```python
from build123d import *

# Parameters (mm, degrees)
F0_W     = 16.6126135737
F0_H     = 3.81
F0_W_2   = 7.62
F0_H_2   = 7.62
F1_DEPTH = 3.175


# Not quite as in the source:
# - a length typed as a fraction of an inch, garbled in the dataset ("3 / 203.2 mm" for 3/8 in), is restored
# - a feature names something its author has since deleted; it is built from what else it names


with BuildPart() as f1:
    # F0 (on Top) → F1 (new body)
    with BuildSketch(Plane.XY):
        Polygon((24.765, -8.001), (41.275, -8.001), (41.275, 19.939), (24.765, 19.939), (24.765, 16.891), (17.907, 16.891), (17.907, 14.351), (19.939, 14.351), (19.939, 11.811), (17.907, 11.811), (17.907, 10.541), (15.113, 10.541), (15.113, 11.811), (13.081, 11.811), (13.081, 14.351), (15.113, 14.351), (15.113, 16.891), (8.255, 16.891), (8.255, 19.939), (-8.255, 19.939), (-8.255, 16.891), (-15.113, 16.891), (-15.113, 14.351), (-13.081, 14.351), (-13.081, 11.811), (-15.113, 11.811), (-15.113, 10.541), (-17.907, 10.541), (-17.907, 11.811), (-19.939, 11.811), (-19.939, 14.351), (-17.907, 14.351), (-17.907, 16.891), (-24.765, 16.891), (-24.765, 19.939), (-41.275, 19.939), (-41.275, -8.001), (-24.765, -8.001), (-24.765, -4.953), (-17.907, -4.953), (-17.907, -2.413), (-19.939, -2.413), (-19.939, 0.127), (-17.907, 0.127), (-17.907, 1.397), (-15.113, 1.397), (-15.113, 0.127), (-13.081, 0.127), (-13.081, -2.413), (-15.113, -2.413), (-15.113, -4.953), (-8.255, -4.953), (-8.255, -8.001), (8.255, -8.001), (8.255, -4.953), (15.113, -4.953), (15.113, -2.413), (13.081, -2.413), (13.081, 0.127), (15.113, 0.127), (15.113, 1.397), (17.907, 1.397), (17.907, 0.127), (19.939, 0.127), (19.939, -2.413), (17.907, -2.413), (17.907, -4.953), (24.765, -4.953), align=None)
        with Locations((0.0095833093, -1.778)):
            Rectangle(F0_W, F0_H, mode=Mode.SUBTRACT)
        with Locations((0, 5.969)):
            Rectangle(F0_W_2, F0_H_2, mode=Mode.SUBTRACT)
    extrude(amount=F1_DEPTH)


solid = f1.part
```
Geometry: final body of the model. Coordinates: model frame, mm. A direction names the side the tool comes from. Coordinates: 2 decimals unless noted, no trailing zeros. Order: outer loops, then holes, each group sorted by start corner. A loop starts at its lowest first (then second) coordinate and runs counter-clockwise, first axis right, second up. Notation, with made-up numbers: (40, 89) - (96, 89) arc R11 cw to (96, 108) - close; hole circle Ø3 at (-18.75, 52.5). An arc over 180 degrees is marked (long way). Return JSON: item names as keys, results as strings. Group by question number.
1. Cut plane A-A (y = 16). Output: boundary loops of the cut face in (x, z) (3 decimals).
2. Cut plane B-B (x = -14). Output: boundary loops of the cut face in (y, z) (3 decimals).
3. Cut plane D-D (y = 6). Output: boundary loops of the cut face in (x, z) (3 decimals).
4. Pin query (flat end, axial travel): pin 1 (0.6 mm diameter, centred on x = -14.5, z = 2, fed in from +Y); pin 2 (0.8 mm diameter, centred on x = 16, z = 1.5, fed in from +Y). Return the tip coordinate at first contact, or that it passes through.
5. Set-up query: faces 1 (the face through (-14, 0.127, 2)), 2 (the face through (33, -8.001, 2)), 3 (the face through (12, -4.953, 2)), 4 (the face through (-8.255, 18, 2)). Return all of +Z, -Z, +X, -X, +Y, -Y with unobstructed straight access to the full face (end or side cutting, diameter ignored); none if empty.
6. Material intervals for line 1 along X through (y, z) = (-1, 0.95) (3 decimals); line 2 along X through (y, z) = (16.5, 2.5) (3 decimals); line 3 along X through (y, z) = (13, 0.3) (3 decimals), sorted ascending. Write a range as [from, to].
7. Pull-direction query (Y, two-part tool) for faces 5 (the face through (-8.255, -6, 2)), 6 (the face through (16, 1.397, 2)), 7 (the face through (-3.81, 6, 2)); classes: pulls with the +Y half, pulls with the -Y half, needs draft (parallel to the pull), parting line crosses it, or undercut.
8. Cut plane C-C (y = -1). Output: boundary loops of the cut face in (x, z) (3 decimals), plus the area to 3 significant figures.
Resolved:
{
 "1": {"outline": "(-41.275, 0) - (-17.907, 0) - (-17.907, 3.175) - (-41.275, 3.175) - close; (-15.113, 0) - (15.113, 0) - (15.113, 3.175) - (-15.113, 3.175) - close; (17.907, 0) - (41.275, 0) - (41.275, 3.175) - (17.907, 3.175) - close"},
 "2": {"outline": "(-4.953, 0) - (-2.413, 0) - (-2.413, 3.175) - (-4.953, 3.175) - close; (0.127, 0) - (11.811, 0) - (11.811, 3.175) - (0.127, 3.175) - close; (14.351, 0) - (16.891, 0) - (16.891, 3.175) - (14.351, 3.175) - close"},
 "3": {"outline": "(-41.275, 0) - (-3.81, 0) - (-3.81, 3.175) - (-41.275, 3.175) - close; (3.81, 0) - (41.275, 0) - (41.275, 3.175) - (3.81, 3.175) - close"},
 "4": {"pin 1": "stops at y = 16.89", "pin 2": "stops at y = 10.54"},
 "5": {"face 1": "+Z, -Z", "face 2": "+Z, -Z, +X, -X, -Y", "face 3": "+Z, -Z, -Y", "face 4": "+Z, -Z, +Y"},
 "6": {"line 1": "x = [-41.275, -19.939], [-13.081, -8.297], [8.316, 13.081], [19.939, 41.275]", "line 2": "x = [-41.275, -17.907], [-15.113, 15.113], [17.907, 41.275]", "line 3": "x = [-41.275, -19.939], [-13.081, 13.081], [19.939, 41.275]"},
 "7": {"face 5": "needs draft", "face 6": "pulls with the -Y half", "face 7": "undercut"},
 "8": {"outline": "(-41.275, 0) - (-19.939, 0) - (-19.939, 3.175) - (-41.275, 3.175) - close; (-13.081, 0) - (-8.297, 0) - (-8.297, 3.175) - (-13.081, 3.175) - close; (8.316, 0) - (13.081, 0) - (13.081, 3.175) - (8.316, 3.175) - close; (19.939, 0) - (41.275, 0) - (41.275, 3.175) - (19.939, 3.175) - close", "area": "166 mm²"}
}
